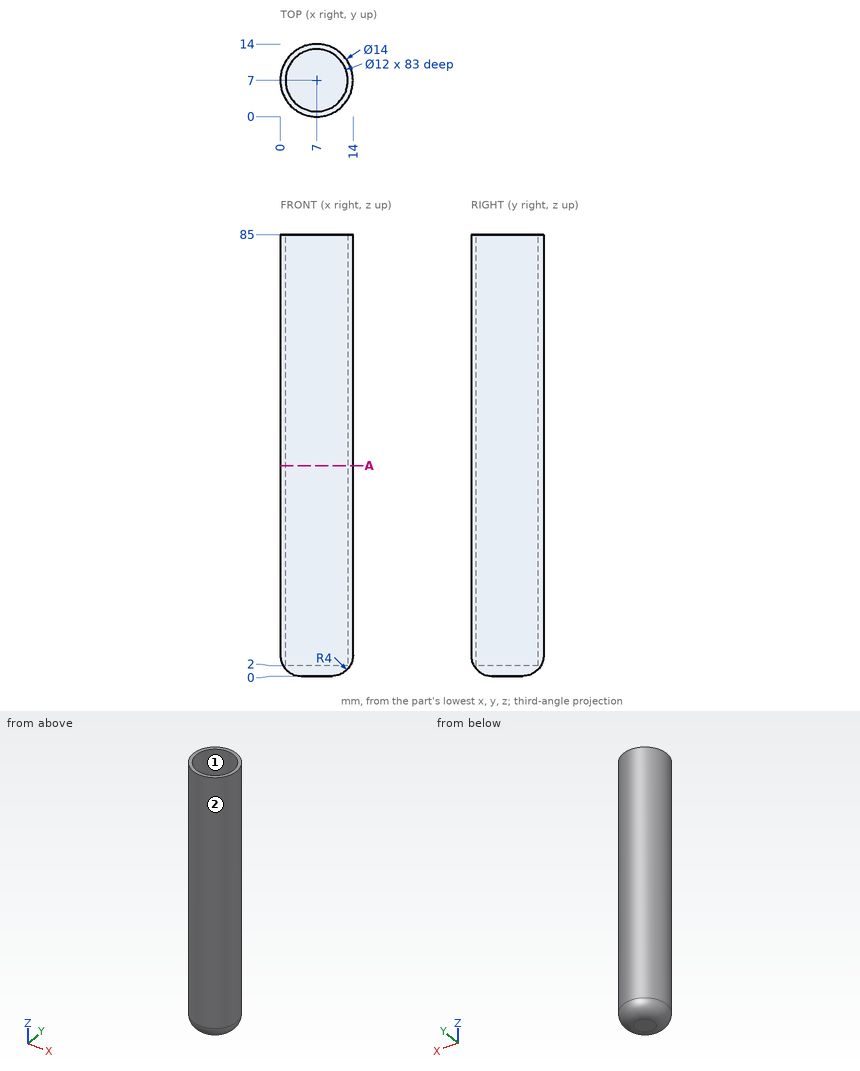
Can you work these out from the drawing? Everything is in mm from the part's minimum corner. Give positions to 0.01 mm unless a question says otherwise; leave off trailing zeros. Loops run counter-clockwise (first coordinate to the right, second up) from the corner with the lowest first, then second, coordinate; pieces in that order, holes last. Notation, with made-up numbers: (65.25, 28) -> (87.25, 28) arc R34 ccw to (87.25, 65) -> close; hole circle Ø10 at (-22.5, 47.25). An arc over 180 degrees is marked (long way). Return JSON: item names as keys, results as strings.
Q1. We'd pull the mould along Y, two halves only. Please class the marked faces 1 and 2: released by +Y, released by -Y, zero draft, split by the parting line, or undercut.
Checks:
{"face 1": "undercut", "face 2": "split by the parting line"}
Q2. I need wall thicknesses on probe 1 along Y at (x, z) = (7, 41.5); probe 2 along Y at (x, z) = (10.75, 15.5); probe 3 along X at (y, z) = (11.5, 62.5). Which ranges of each line are inside material? Lowest first, please.
Checks:
{"probe 1": "y = 0 to 1, 13 to 14", "probe 2": "y = 1.09 to 2.32, 11.68 to 12.91", "probe 3": "x = 1.64 to 3.03, 10.97 to 12.36"}
Q3. For pin 1 Ø1.5 at (y, z) = (8, 41.5) entering from -X; pin 2 Ø3.5 at (x, y) = (7.5, 6) entering from +Z, each with a flat end and sliding along its axis, tell me the tip position at first contact or that it passes through.
Checks:
{"pin 1": "stops at x = 0", "pin 2": "stops at z = 2"}
Q4. I want a section at A-A, the plane z = 40.5. List the corners of the cut face in (x, y) for me, then the cut area to 3 significant figures.
Checks:
{"outline": "circle Ø14 at (7, 7); hole circle Ø12 at (7, 7)", "area": "40.8 mm2"}
